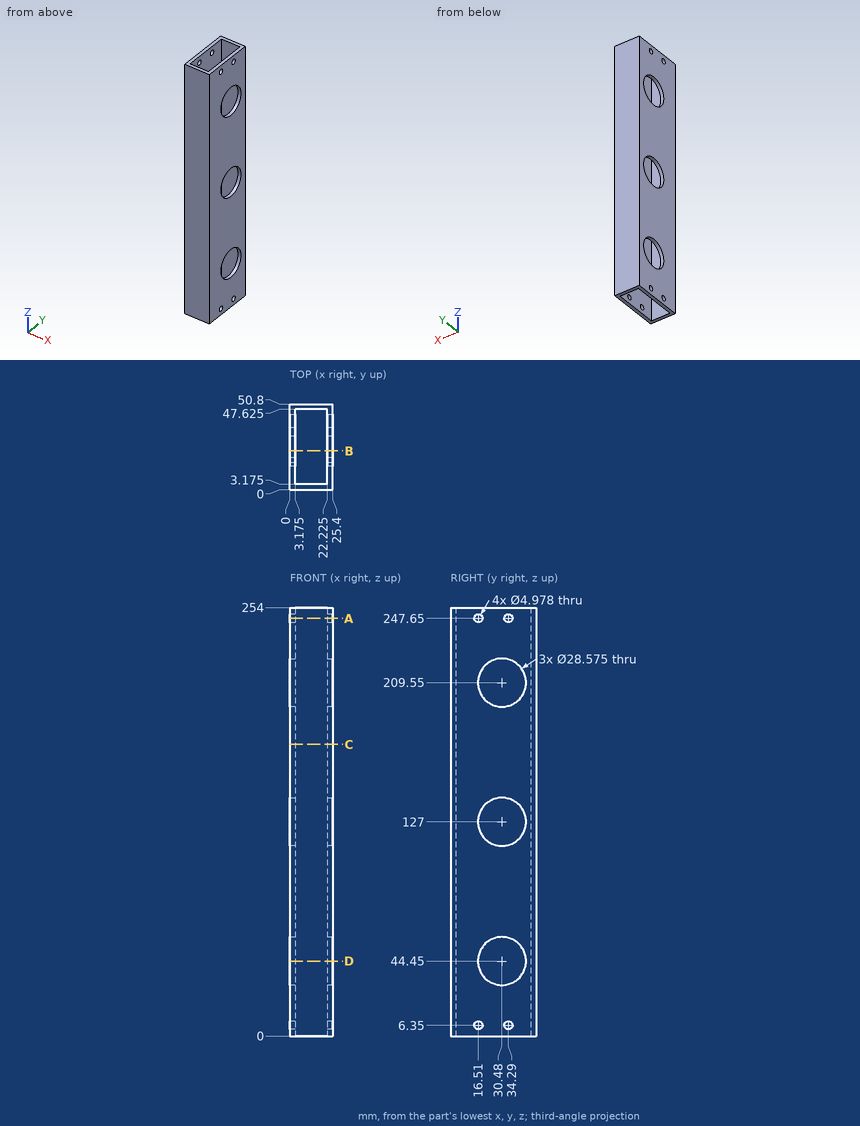
Design review of the part shown in the three views and the two pictorial views. Dimensions are in mm from the part's minimum x, y and z. Coordinates: 2 decimals unless noted, no trailing zeros. Loops run counter-clockwise (first coordinate to the right, second up) from the corner with the lowest first, then second, coordinate; pieces in that order, holes last.
(1) Consider section A-A, the plane z = 247.65. Give the boundary of the cut face in (x, y) (1 decimal).
Determined:
outline: (0, 0) - (25.4, 0) - (25.4, 14) - (22.2, 14) - (22.2, 3.2) - (3.2, 3.2) - (3.2, 14) - (0, 14) - close; (0, 19) - (3.2, 19) - (3.2, 31.8) - (0, 31.8) - close; (0, 36.8) - (3.2, 36.8) - (3.2, 47.6) - (22.2, 47.6) - (22.2, 36.8) - (25.4, 36.8) - (25.4, 50.8) - (0, 50.8) - close; (22.2, 19) - (25.4, 19) - (25.4, 31.8) - (22.2, 31.8) - close
(2) Consider section C-C, the plane z = 173. Give the boundary of the cut face in (x, y) (1 decimal).
Determined:
outline: (0, 0) - (25.4, 0) - (25.4, 50.8) - (0, 50.8) - close; hole (3.2, 3.2) - (22.2, 3.2) - (22.2, 47.6) - (3.2, 47.6) - close
(3) Consider section D-D, the plane z = 44.45. Give the boundary of the cut face in (x, y) (1 decimal).
Determined:
outline: (0, 0) - (25.4, 0) - (25.4, 16.2) - (22.2, 16.2) - (22.2, 3.2) - (3.2, 3.2) - (3.2, 16.2) - (0, 16.2) - close; (0, 44.8) - (3.2, 44.8) - (3.2, 47.6) - (22.2, 47.6) - (22.2, 44.8) - (25.4, 44.8) - (25.4, 50.8) - (0, 50.8) - close
(4) Wall thickness on L1, parallel to Z at x = 24, y = 30; L2, parallel to Y at x = 1.8, z = 247.65; L3, parallel to Y at x = 13.25, z = 108.5 (1 decimal): over which ranges is each line inside the solid? List them lowest first.
Determined:
L1: z = 0 to 30.17, 58.73 to 112.72, 141.28 to 195.27, 223.83 to 254
L2: y = 0 to 14.02, 19 to 31.8, 36.78 to 50.8
L3: y = 0 to 3.2, 47.6 to 50.8
(5) Consider section B-B, the plane y = 23. Give the number of separate pieces and of enclosed holes in the cut face, plus the area to 3 significant figures.
Determined:
separate pieces: 8
enclosed holes: 0
area: 1,150 mm2
